Verification items for the finished model (mm, model axes). Face numbers are marked on the shaded views. A direction names the side the tool comes from. Give positions to 0.01 mm unless a question says otherwise; leave off trailing zeros. Loops run counter-clockwise (first coordinate to the right, second up) from the corner with the lowest first, then second, coordinate; pieces in that order, holes last. Notation, with made-up numbers: M -35.75,-28.75 L 8.25,-28.75 A18 cw 8.25,-19.75 Z; hole C 9.5,-28 d4. An arc over 180 degrees is marked long. Answer in a Markdown table with one row per item.
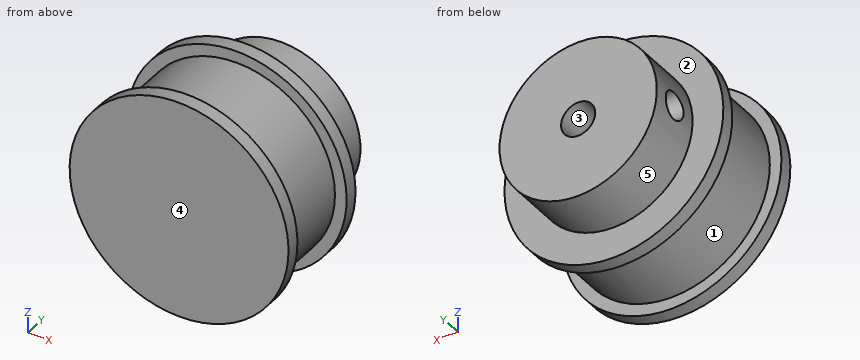
```python
from build123d import *

# Parameters (mm, degrees)
SKETCH_1_R          = 11.5
SKETCH_1_R_2        = 2.5
EXTRUDE_1_DEPTH     = 8
SKETCH_2_R          = 16
EXTRUDE_2_DEPTH     = 2
SKETCH_3_R          = 14.3
EXTRUDE_3_DEPTH     = 11
SKETCH_4_R          = 16
EXTRUDE_4_DEPTH     = 2
SKETCH_5_R          = 2
CUT_EXTRUDE_1_DEPTH = 19


with BuildPart() as part:
    # 草图1 → 凸台-拉伸1 (new body)
    with BuildSketch(Plane(origin=(0, 0, 0), x_dir=(1, 0, 0), z_dir=(0, 1, 0))):
        with Locations(Location((0, 0, 0), (0, 0, 270))):
            Circle(SKETCH_1_R)
        with Locations(Location((0, 0, 0), (0, 0, 270))):
            Circle(SKETCH_1_R_2, mode=Mode.SUBTRACT)
    extrude(amount=EXTRUDE_1_DEPTH)

    # 草图2 → 凸台-拉伸2 (add)
    with BuildSketch(Plane.XZ):
        with Locations(Location((0, 0, 0), (0, 0, 270))):
            Circle(SKETCH_2_R)
    extrude(amount=EXTRUDE_2_DEPTH)

    # 草图3 → 凸台-拉伸3 (add)
    with BuildSketch(Plane.XZ.offset(2)):
        with Locations(Location((0, 0, 0), (0, 0, 270))):
            Circle(SKETCH_3_R)
    extrude(amount=EXTRUDE_3_DEPTH)

    # 草图4 → 凸台-拉伸4 (add)
    with BuildSketch(Plane.XZ.offset(13)):
        with Locations(Location((0, 0, 0), (0, 0, 270))):
            Circle(SKETCH_4_R)
    extrude(amount=EXTRUDE_4_DEPTH)

    # 草图5 → 切除-拉伸1 (cut)
    with BuildSketch(Plane(origin=(0, 0, 0), x_dir=(0, 0, -1), z_dir=(1, 0, 0))):
        with Locations((0, 4)):
            Circle(SKETCH_5_R)
    extrude(amount=-CUT_EXTRUDE_1_DEPTH, mode=Mode.SUBTRACT)


solid = part.part
```
Item 1: Sectioned sample at A-A (z = 0). Record the cut outline in (x, y).
Reported:
| item | result |
|---|---|
| outline | M -16,-15 L 16,-15 L 16,-13 L 14.3,-13 L 14.3,-2 L 16,-2 L 16,0 L 11.5,0 L 11.5,8 L 2.5,8 L 2.5,0 L -2.5,0 L -2.5,2 L -11.5,2 L -11.5,0 L -16,0 L -16,-2 L -14.3,-2 L -14.3,-13 L -16,-13 Z; M -11.5,6 L -2.5,6 L -2.5,8 L -11.5,8 Z |
Item 2: Sectioned sample at B-B (x = -7.5). Record the cut outline in (y, z), and give its area (3 significant figures).
Reported:
| item | result |
|---|---|
| outline | M -15,-14.13 L -13,-14.13 L -13,-12.18 L -2,-12.18 L -2,-14.13 L 0,-14.13 L 0,-8.72 L 8,-8.72 L 8,8.72 L 0,8.72 L 0,14.13 L -2,14.13 L -2,12.18 L -13,12.18 L -13,14.13 L -15,14.13 Z; hole C 4,0 d4 |
| area | 508 mm^2 |
Item 3: Release check for a two-part mould opening along X. For the marked faces 1, 2 and 3 record: released by +X, released by -X, zero draft, split by the parting line, or undercut.
Reported:
| item | result |
|---|---|
| face 1 | split by the parting line |
| face 2 | zero draft |
| face 3 | undercut |
Item 4: Sectioned sample at D-D (z = -7). Record the cut outline in (x, y).
Reported:
| item | result |
|---|---|
| outline | M -14.39,-15 L 14.39,-15 L 14.39,-13 L 12.47,-13 L 12.47,-2 L 14.39,-2 L 14.39,0 L 9.12,0 L 9.12,8 L -9.12,8 L -9.12,0 L -14.39,0 L -14.39,-2 L -12.47,-2 L -12.47,-13 L -14.39,-13 Z |
Item 5: Go/stop test with flat-tipped pins: pin 1 (10 mm diameter, centred on y = 0.5, z = 9, fed in from -X); pin 2 (4.5 mm diameter, centred on y = 4, z = 0, fed in from +X); pin 3 (1.5 mm diameter, centred on x = 9, y = 1.5, fed in from +Z). Record where each tip stops, or that it passes through.
Reported:
| item | result |
|---|---|
| pin 1 | stops at x = -15.49 |
| pin 2 | stops at x = 11.5 |
| pin 3 | stops at z = 8.01 |
Item 6: Sectioned sample at C-C (x = 0). Record the cut outline in (y, z).
Reported:
| item | result |
|---|---|
| outline | M -15,-16 L -13,-16 L -13,-14.3 L -2,-14.3 L -2,-16 L 0,-16 L 0,-11.5 L 8,-11.5 L 8,-2.5 L 0,-2.5 L 0,2.5 L 8,2.5 L 8,11.5 L 0,11.5 L 0,16 L -2,16 L -2,14.3 L -13,14.3 L -13,16 L -15,16 Z |
Item 7: Scan lines: L1, parallel to Y at x = -10.5, z = 10.5; L2, parallel to Y at x = -4.5, z = 0; L3, parallel to Y at x = -12.5, z = -3. Record each from-to range of solid material in increasing order. Write a range as [from, to].
Reported:
| item | result |
|---|---|
| L1 | y = [-15, -13], [-2, 0] |
| L2 | y = [-15, 2], [6, 8] |
| L3 | y = [-15, 0] |
Item 8: Tool access check on the marked faces 4 and 5. Record the directions out of +Z, -Z, +X, -X, +Y, -Y that give a thin tool (end or side, any length) a straight path to the whole face; none if there is none.
Reported:
| item | result |
|---|---|
| face 4 | +Z, -Z, +X, -X, -Y |
| face 5 | +Y |
